The drawing under review shows one solid part. Ordinate dimensions are in mm from its lowest x, y, z. A direction names the side the tool comes from. Give positions to 0.01 mm unless a question says otherwise; leave off trailing zeros. Loops run counter-clockwise (first coordinate to the right, second up) from the corner with the lowest first, then second, coordinate; pieces in that order, holes last.
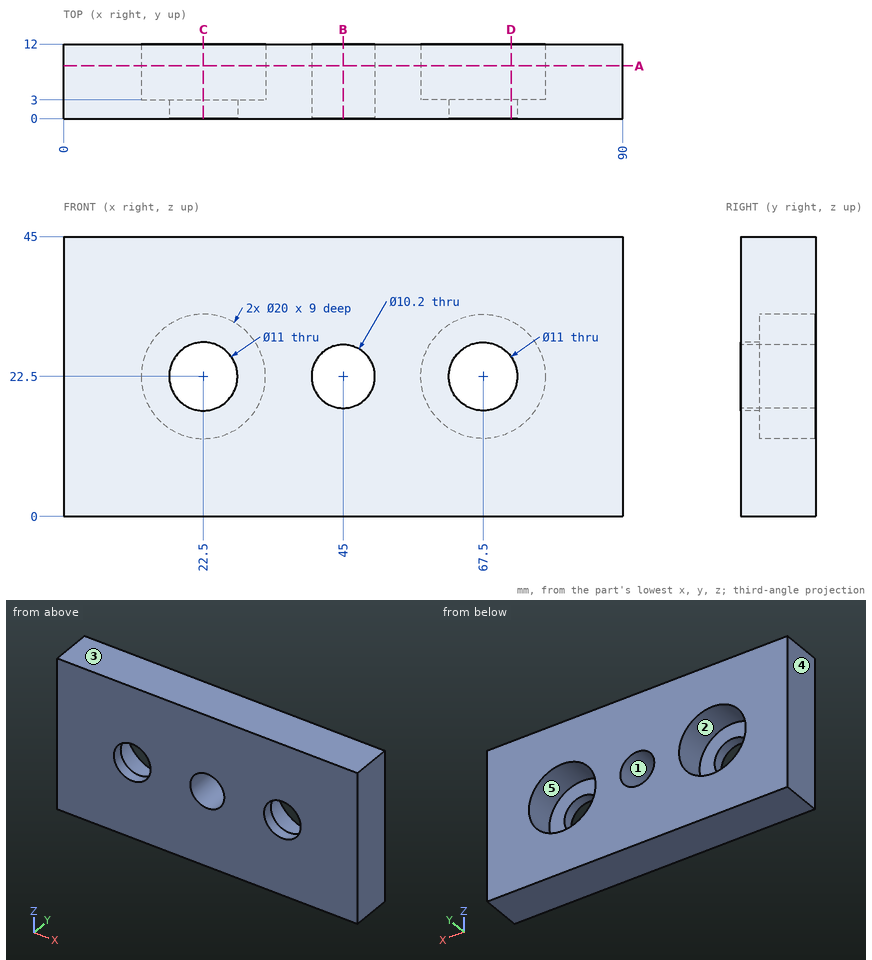
Item 1: Tool access review of the marked faces 1 and 2: name each direction out of +Z, -Z, +X, -X, +Y, -Y from which nothing blocks a thin tool from reaching the whole face with its end or side.
Answer:
face 1: +Y, -Y
face 2: +Y
Item 2: The part is to be moulded in two halves that separate along X. For the marked faces 3, 4 and 5, say which applies: released by +X, released by -X, zero draft, split by the parting line, or undercut.
Answer:
face 3: zero draft
face 4: released by -X
face 5: undercut
Item 3: Take a section at B-B on x = 45. Give the boundary of the cut face in (y, z), and give its area (3 significant figures).
Answer:
outline: (0, 0) - (12, 0) - (12, 17.4) - (0, 17.4) - close; (0, 27.6) - (12, 27.6) - (12, 45) - (0, 45) - close
area: 418 mm2
Item 4: Take a section at D-D on x = 72. Give the boundary of the cut face in (y, z).
Answer:
outline: (0, 0) - (12, 0) - (12, 13.57) - (3, 13.57) - (3, 19.34) - (0, 19.34) - close; (0, 25.66) - (3, 25.66) - (3, 31.43) - (12, 31.43) - (12, 45) - (0, 45) - close
Item 5: Clearance check with flat-ended pins moving along their axes: pin 1 Ø6 at (x, z) = (45, 22.5) entering from -Y; pin 2 Ø6 at (x, z) = (63.5, 21) entering from +Y. State where each tip first meets the part, or that it passes through.
Answer:
pin 1: passes through
pin 2: stops at y = 3
Item 6: Take a section at C-C on x = 22.5. Give the boundary of the cut face in (y, z).
Answer:
outline: (0, 0) - (12, 0) - (12, 12.5) - (3, 12.5) - (3, 17) - (0, 17) - close; (0, 28) - (3, 28) - (3, 32.5) - (12, 32.5) - (12, 45) - (0, 45) - close
Item 7: For L1, parallel to X at y = 7.5, z = 22.5; L2, parallel to X at y = 2.15, z = 22.5; L3, parallel to Z at x = 67.5, y = 6.5, list the stretches that pass through material, from the lowest coordinate up.
Answer:
L1: x = 0 to 12.5, 32.5 to 39.9, 50.1 to 57.5, 77.5 to 90
L2: x = 0 to 17, 28 to 39.9, 50.1 to 62, 73 to 90
L3: z = 0 to 12.5, 32.5 to 45
Item 8: Take a section at A-A on y = 8.5. Give the boundary of the cut face in (x, z), and give its area (3 significant figures).
Answer:
outline: (0, 0) - (90, 0) - (90, 45) - (0, 45) - close; hole circle Ø20 at (22.5, 22.5); hole circle Ø10.2 at (45, 22.5); hole circle Ø20 at (67.5, 22.5)
area: 3,340 mm2
